Check sheet for the modelled part. Datum: model origin and axes. Units: mm. A direction names the side the tool comes from. Round coordinates to 2 decimals unless told otherwise and drop trailing zeros. Write each loop counter-clockwise with the first axis right and the second up, starting at its lowest first coordinate (ties: lowest second). Pieces come first, ordered by that corner, then holes. Notation, with made-up numbers: M 48.25,-27 L 95.25,-27 A19 cw 95.25,-12 Z; hole C 26,12 d6. An arc over 180 degrees is marked long. Put each result on its own line as item: value.
```python
from build123d import *

# Parameters (mm, degrees)
F1_DEPTH = 5
F2_W     = 5
F2_H     = 40
F3_DEPTH = 12
F4_R     = 3
F5_R     = 1.5
F6_DEPTH = 10


with BuildPart() as f1:
    # F0 (on Top) → F1 (new body)
    with BuildSketch(Plane.XY):
        with BuildLine():
            ThreePointArc((-8.809511, 7.392058), (11.5, 0), (-8.809511, -7.392058))
            Line((-8.809511, -7.392058), (-14.94391, -7.392058))
            ThreePointArc((-14.94391, -7.392058), (-15.806941, -7.886907), (-15.815832, -8.881703))
            ThreePointArc((-15.815832, -8.881703), (-14.920363, -10.315422), (-13.895319, -11.659557))
            ThreePointArc((-13.895319, -11.659557), (2.827372, -17.917342), (16.810487, -6.814154))
            ThreePointArc((16.810487, -6.814154), (18.174589, -6.14164), (19.677769, -5.910335))
            Line((19.677769, -5.910335), (30.5, -5.910335))
            ThreePointArc((30.5, -5.910335), (34.035534, -7.374801), (35.5, -10.910335))
            Line((35.5, -10.910335), (35.5, -18))
            ThreePointArc((35.5, -18), (36.085786, -19.414214), (37.5, -20))
            Line((37.5, -20), (45.5, -20))
            Line((45.5, -20), (45.5, 0))
            Line((45.5, 0), (45.5, 20))
            Line((45.5, 20), (37.5, 20))
            ThreePointArc((37.5, 20), (36.085786, 19.414214), (35.5, 18))
            Line((35.5, 18), (35.5, 10.910335))
            ThreePointArc((35.5, 10.910335), (34.035534, 7.374801), (30.5, 5.910335))
            Line((30.5, 5.910335), (19.677769, 5.910335))
            ThreePointArc((19.677769, 5.910335), (18.174589, 6.14164), (16.810487, 6.814154))
            ThreePointArc((16.810487, 6.814154), (2.827372, 17.917342), (-13.895319, 11.659557))
            ThreePointArc((-13.895319, 11.659557), (-14.920363, 10.315422), (-15.815832, 8.881703))
            ThreePointArc((-15.815832, 8.881703), (-15.806941, 7.886907), (-14.94391, 7.392058))
            Line((-14.94391, 7.392058), (-8.809511, 7.392058))
        make_face()
    extrude(amount=F1_DEPTH)

    # F2 (on face) → F3 (join)
    with BuildSketch(Plane.XY.offset(5)):
        with Locations((43, 0)):
            Rectangle(F2_W, F2_H)
    extrude(amount=F3_DEPTH)

    # F4
    f4_edges = [f1.edges().sort_by_distance(p)[0] for p in [
        (40.5, 0, 5),
        (43, 20, 17),
        (43, -20, 17),
    ]]
    fillet(f4_edges, radius=F4_R)

    # F5 (on face) → F6 (cut)
    with BuildSketch(Plane(origin=(40.5, 0, 0), x_dir=(0, -1, 0), z_dir=(-1, 0, 0))):
        with Locations((-11.877556, 12)):
            Circle(F5_R)
        with Locations((11.877556, 12)):
            Circle(F5_R)
    extrude(amount=-F6_DEPTH, mode=Mode.SUBTRACT)


solid = f1.part
```
1. Cross-section at A-A (z = 12). Enter the section's corners in (x, y).
Computed values:
outline: M 40.5,-20 L 45.5,-20 L 45.5,-13.38 L 40.5,-13.38 Z; M 40.5,-10.38 L 45.5,-10.38 L 45.5,10.38 L 40.5,10.38 Z; M 40.5,13.38 L 45.5,13.38 L 45.5,20 L 40.5,20 Z
2. Depth check by flat-ended pin: pin 1 Ø2.5 at (y, z) = (15.5, 2) entering from -X; pin 2 Ø12 at (x, y) = (29, -9) entering from -Z; pin 3 Ø2 at (x, z) = (38, 13) entering from +Y; pin 4 Ø1.5 at (y, z) = (-16, 2) entering from -X. Enter the tip coordinate at first touch or a pass-through.
Computed values:
pin 1: stops at x = -11.22
pin 2: stops at z = 0
pin 3: passes through
pin 4: stops at x = -9.82
3. Cross-section at C-C (y = 0). Enter the section's corners in (x, z), then the cut area to 3 significant figures.
Computed values:
outline: M 11.5,0 L 45.5,0 L 45.5,17 L 40.5,17 L 40.5,8 A3 cw 37.5,5 L 11.5,5 Z
area: 232 mm2
4. Scan lines: probe 1 along Y at (x, z) = (0, 1.65); probe 2 along X at (y, z) = (8, 1.5); probe 3 along Z at (x, y) = (33, -3). Record each from-to range of solid material in increasing order.
Computed values:
probe 1: y = -18.14 to -11.5, 11.5 to 18.14
probe 2: x = -15.86 to -8.26, 8.26 to 16.28, 34.57 to 45.5
probe 3: z = 0 to 5
5. Cross-section at D-D (y = 4.5). Enter the section's corners in (x, z).
Computed values:
outline: M 10.58,0 L 45.5,0 L 45.5,17 L 40.5,17 L 40.5,8 A3 cw 37.5,5 L 10.58,5 Z
6. Cross-section at B-B (x = 0). Enter the section's corners in (y, z).
Computed values:
outline: M -18.14,0 L -11.5,0 L -11.5,5 L -18.14,5 Z; M 11.5,0 L 18.14,0 L 18.14,5 L 11.5,5 Z
7. Access from +Z, -Z, +X, -X, +Y, -Y to the whole of each face (thin tool, end or side, straight path). Record for faces 4 (the cylindrical face through (34, -7.34, 2.46)), 5 (the flat face through (35.5, 15, 2)), 6 (the flat face through (13, 0, 5)).
Computed values:
face 4: +Z, -Z, -Y
face 5: +Z, -Z, +Y
face 6: +Z, -X, +Y, -Y
8. Release check for a two-part mould opening along Y. For faces 1 (the cylindrical face through (43.04, 19.1, 16.14)), 2 (the flat face through (42, -20, 7)), 3 (the flat face through (-12, 7.392, 2)) record: +Y half, -Y half, draft (parallel to the pull), parting line (faces both ways), or undercut.
Computed values:
face 1: +Y half
face 2: -Y half
face 3: undercut
